from build123d import *

# Parameters (mm, degrees)
SKETCH3_R            = 1.5
FIXATION_HOLES_DEPTH = 80.101201002
SKETCH4_R            = 1.5
SHAFT_DEPTH          = 6


with BuildPart() as part:
    # Sketch2 → Body (revolve)
    with BuildSketch(Plane(origin=(0, 0, 0), x_dir=(0, 0, -1), z_dir=(1, 0, 0)), mode=Mode.PRIVATE) as body_sk:
        with BuildLine():
            Line((0, 0), (0, 32))
            ThreePointArc((0, 32), (-5.149715015, 41.518162483), (-15, 46))
            Line((-15, 46), (-32.5, 46))
            Line((-32.5, 46), (-32.5, 42))
            Line((-32.5, 42), (-15, 42))
            ThreePointArc((-15, 42), (-8.566932971, 38.739760326), (-6, 32))
            Line((-6, 32), (-6, 10))
            Line((-6, 10), (-45, 10))
            Line((-45, 10), (-45, 0))
            Line((-45, 0), (0, 0))
        make_face()
    revolve(body_sk.sketch.rotate(Axis((0, 0, 677.96312991), (0, 0, -1)), 90), axis=Axis((0, 0, 677.96312991), (0, 0, -1)))

    # Sketch3 → Fixation_Holes (cut, through all)
    with BuildSketch(Plane(origin=(0, 0, 0), x_dir=(-1, 0, 0), z_dir=(0, 0, -1))):
        with Locations((-11.25, 11.25)):
            Circle(SKETCH3_R)
        with Locations((11.25, 11.25)):
            Circle(SKETCH3_R)
        with Locations((11.25, -11.25)):
            Circle(SKETCH3_R)
        with Locations((-11.25, -11.25)):
            Circle(SKETCH3_R)
    extrude(amount=-FIXATION_HOLES_DEPTH, mode=Mode.SUBTRACT)

    # Sketch4 → Shaft (add)
    with BuildSketch(Plane(origin=(0, 0, 0), x_dir=(-1, 0, 0), z_dir=(0, 0, -1))):
        with Locations(Location((0, 0, 0), (0, 0, 180))):
            Circle(SKETCH4_R)
    extrude(amount=SHAFT_DEPTH)


solid = part.part
Model file for the job. Use its own axes, mm. A direction names the side the tool comes from. Coordinates: 2 decimals unless noted, no trailing zeros. Write each loop counter-clockwise with the first axis right and the second up, starting at its lowest first coordinate (ties: lowest second). Pieces come first, ordered by that corner, then holes. Notation, with made-up numbers: (64, -19.5) -> (104, -19.5) arc R18 cw to (104, -0.5) -> close; hole circle Ø6 at (4.25, -8). An arc over 180 degrees is marked (long way). One line per item, written item: value. Start each with the question number.
1) Pull direction X, two halves, no side cores. Call faces 4 (the face through (0, 0, -6)), 5 (the face through (-5.99, -45.61, 23.87)), 6 (the face through (-8, 7, 6)): +X half, -X half, draft (parallel to the pull), parting line (faces both ways), or undercut.
2) Which spindle directions (+Z, -Z, +X, -X, +Y, -Y) get a long thin tool onto all of the face, cutting with end or side? Do faces 1 (the face through (40.06, -12.62, 23.63)), 2 (the face through (1.43, -0.45, -2.96)), 3 (the face through (-9.75, 11.32, 2.96)). Say none if no direction does.
3) Slice it at A-A on x = 0. Write the cut outline in (y, z).
4) Slice it at D-D on x = -11.25. Count the separate pieces of the cut face and the enclosed holes in it, then the cut area to 3 significant figures.
5) Probe probe 1 along Y at (x, z) = (11, 2); probe 2 along X at (y, z) = (-6.5, 14); probe 3 along X at (y, z) = (-6, 13). List the from-to ranges inside material, lowest first.
6) Flat gauge pins, fed straight in: pin 1 Ø4 at (x, y) = (11.25, -11.25) entering from -Z; pin 2 Ø5 at (x, z) = (-35.5, 13.5) entering from +Y; pin 3 Ø5 at (x, y) = (34, -30.5) entering from -Z; pin 4 Ø1.5 at (y, z) = (-28.5, 34.5) entering from +X. Where does each tip first touch, or does it go through?
7) Slice it at C-C on z = 4.5. Write the cut outline in (x, y).
Answers follow:
1. face 4: draft
1. face 5: parting line
1. face 6: undercut
2. face 1: +Z
2. face 2: -Z
2. face 3: +Z, -Z
3. outline: (-46, 15) arc R17 ccw to (-32, 0) -> (-1.5, 0) -> (-1.5, -6) -> (1.5, -6) -> (1.5, 0) -> (32, 0) arc R17 ccw to (46, 15) -> (46, 32.5) -> (42, 32.5) -> (42, 15) arc R10 cw to (32, 6) -> (10, 6) -> (10, 45) -> (-10, 45) -> (-10, 6) -> (-32, 6) arc R10 cw to (-42, 15) -> (-42, 32.5) -> (-46, 32.5) -> close
4. separate pieces: 3
4. enclosed holes: 0
4. area: 644 mm2
5. probe 1: -35.9 to -12.73, -9.77 to 9.77, 12.73 to 35.9
5. probe 2: -45.4 to -41.34, -7.6 to 7.6, 41.34 to 45.4
5. probe 3: -45.28 to -41.15, -8 to 8, 41.15 to 45.28
6. pin 1: z = 0
6. pin 2: y = 31.8
6. pin 3: z = 7.23
6. pin 4: through
7. outline: circle Ø81.76 at (0, 0); hole circle Ø3 at (-11.25, -11.25); hole circle Ø3 at (-11.25, 11.25); hole circle Ø3 at (11.25, -11.25); hole circle Ø3 at (11.25, 11.25)
